Input: part model. Units: mm. Frame: model coordinates. A direction names the side the tool comes from. Round coordinates to 2 decimals unless told otherwise and drop trailing zeros. Loops run counter-clockwise (first coordinate to the right, second up) from the corner with the lowest first, then second, coordinate; pieces in that order, holes last. Notation, with made-up numbers: M 40,45.25 L 52,45.25 A21 ccw 52,84.25 Z; hole C 67,9 d9. An arc over 180 degrees is marked long. Use one line per item in the form item = value. Start each with the question number.
Q1. Section query A-A, the plane x = 0. Output: boundary loops of the cut face in (y, z).
Q2. Section query B-B, the plane z = -44. Output: boundary loops of the cut face in (x, y).
Q3. Section query C-C, the plane x = -18. Output: boundary loops of the cut face in (y, z), and give its area (3 significant figures).
Q4. Access query for faces 1 (the conical face through (64.135, 13.608, -12.544)), 2 (the cylindrical face through (-63.014, 56.359, -12.703)), 3 (the conical face through (61.865, 13.608, -12.544)). Directions: +Z, -Z, +X, -X, +Y, -Y. A direction counts if a zero-diameter tool reaches every point of the face in a straight line with its end or side. Return the directions, or none.
Q5. Section query D-D, the plane x = -33. Output: boundary loops of the cut face in (y, z).
Q6. Mould query, pull axis Z, two halves, no side actions, for faces 4 (the flat face through (-64.5, 35, -43)), 5 (the cylindrical face through (63.02, 17.77, -65.95)), 6 (the conical face through (64.358, 10.775, -72.764)). Classes: pulls with the +Z half, pulls with the -Z half, needs draft (parallel to the pull), parting line crosses it, or undercut.
Q7. Ray query, line 1 along Y through (x, z) = (18, -1); line 2 along X through (y, z) = (45, -48); line 3 along Y through (x, z) = (62, -38). Return the intervals inside material, ascending.
Q8. First-contact query: P1, Ø2.5, axis at y = 52.32, z = -68, coming from the +X side; P2, Ø1, axis at x = 63, y = 39.5, coming from the -Z side; P3, Ø2, axis at x = 63, y = 37, coming from the +Z side; P4, Ø2.5, axis at x = 0, y = 17, coming from the -Z side. Flat tips, straight axial feed; report the tip coordinate or a pass-through.
```python
from build123d import *

# Parameters (mm, degrees)
F_70MM_DEPTH            = 70
FILLET_1_R              = 3
CUT_EXTRUDE_1_REACH     = 170.612
SKETCH_2_R              = 2.05
SKETCH_2_R_2            = 7.5
CUT_EXTRUDE_2_REACH     = 170.612
SKETCH_3_R              = 9.5
SKETCH_4_W              = 18
SKETCH_4_H              = 45
CUT_EXTRUDE_3_DEPTH     = 169.611980594
FILLET_2_R              = 4
FILLET_3_R              = 35
HOLE_WIZARD_3_1_3_1_1_D = 3.1
CHAMFER_1_SIZE          = 0.5


with BuildPart() as part:
    # 草图1 → 宽70mm (new body)
    with BuildSketch(Plane(origin=(0, 0, 0), x_dir=(1, 0, 0), z_dir=(0, 1, 0))):
        Polygon((-64.5, 0), (64.5, 0), (64.5, 83), (61.5, 83), (61.5, 3), (-61.5, 3), (-61.5, 83), (-64.5, 83), align=None)
    extrude(amount=F_70MM_DEPTH)

    # 圆角1
    fillet_1_edges = [part.edges().sort_by_distance(p)[0] for p in [
        (64.5, 35, 0),
        (-64.5, 35, 0),
        (-61.5, 35, -3),
        (61.5, 35, -3),
    ]]
    fillet(fillet_1_edges, radius=FILLET_1_R)

    # 草图2 → 切除-拉伸1 (cut, up to next)
    with BuildSketch(Plane(origin=(64.5, 0, 0), x_dir=(0, 0, -1), z_dir=(1, 0, 0)), mode=Mode.PRIVATE) as cut_extrude_1_sk1:
        with Locations((38, 35)):
            Circle(SKETCH_2_R)
    cut_extrude_1_tool1 = extrude(cut_extrude_1_sk1.sketch, amount=-CUT_EXTRUDE_1_REACH, mode=Mode.PRIVATE) & part.part
    # 草图2 → 切除-拉伸1 (cut, up to next)
    with BuildSketch(Plane(origin=(64.5, 0, 0), x_dir=(0, 0, -1), z_dir=(1, 0, 0)), mode=Mode.PRIVATE) as cut_extrude_1_sk2:
        with Locations((68, 52.320508076)):
            Circle(SKETCH_2_R)
    cut_extrude_1_tool2 = extrude(cut_extrude_1_sk2.sketch, amount=-CUT_EXTRUDE_1_REACH, mode=Mode.PRIVATE) & part.part
    # 草图2 → 切除-拉伸1 (cut, up to next)
    with BuildSketch(Plane(origin=(64.5, 0, 0), x_dir=(0, 0, -1), z_dir=(1, 0, 0)), mode=Mode.PRIVATE) as cut_extrude_1_sk3:
        with Locations((68, 17.679491924)):
            Circle(SKETCH_2_R)
    cut_extrude_1_tool3 = extrude(cut_extrude_1_sk3.sketch, amount=-CUT_EXTRUDE_1_REACH, mode=Mode.PRIVATE) & part.part
    # 草图2 → 切除-拉伸1 (cut, up to next)
    with BuildSketch(Plane(origin=(64.5, 0, 0), x_dir=(0, 0, -1), z_dir=(1, 0, 0)), mode=Mode.PRIVATE) as cut_extrude_1_sk4:
        with Locations((58, 35)):
            Circle(SKETCH_2_R_2)
    cut_extrude_1_tool4 = extrude(cut_extrude_1_sk4.sketch, amount=-CUT_EXTRUDE_1_REACH, mode=Mode.PRIVATE) & part.part
    add(cut_extrude_1_tool1.solids().sort_by_distance((64.5, 35, -38))[0], mode=Mode.SUBTRACT)
    add(cut_extrude_1_tool2.solids().sort_by_distance((64.5, 52.320508, -68))[0], mode=Mode.SUBTRACT)
    add(cut_extrude_1_tool3.solids().sort_by_distance((64.5, 17.679492, -68))[0], mode=Mode.SUBTRACT)
    add(cut_extrude_1_tool4.solids().sort_by_distance((64.5, 35, -58))[0], mode=Mode.SUBTRACT)

    # 草图3 → 切除-拉伸2 (cut, up to next)
    with BuildSketch(Plane.ZY.offset(64.5), mode=Mode.PRIVATE) as cut_extrude_2_sk1:
        with Locations((-58, 35)):
            Circle(SKETCH_3_R)
    cut_extrude_2_tool1 = extrude(cut_extrude_2_sk1.sketch, amount=-CUT_EXTRUDE_2_REACH, mode=Mode.PRIVATE) & part.part
    add(cut_extrude_2_tool1.solids().sort_by_distance((-64.5, 35, -58))[0], mode=Mode.SUBTRACT)

    # 草图4 → 切除-拉伸3 (cut, through all)
    with BuildSketch(Plane(origin=(64.5, 0, 0), x_dir=(0, 0, -1), z_dir=(1, 0, 0))):
        with Locations((20.5, 35)):
            Rectangle(SKETCH_4_W, SKETCH_4_H)
    extrude(amount=-CUT_EXTRUDE_3_DEPTH, mode=Mode.SUBTRACT)

    # 圆角2
    fillet_2_edges = [part.edges().sort_by_distance(p)[0] for p in [
        (63, 57.5, -29.5),
        (-63, 57.5, -29.5),
        (63, 12.5, -29.5),
        (-63, 12.5, -29.5),
        (63, 12.5, -11.5),
        (-63, 12.5, -11.5),
        (63, 57.5, -11.5),
        (-63, 57.5, -11.5),
    ]]
    fillet(fillet_2_edges, radius=FILLET_2_R)

    # 圆角3
    fillet_3_edges = [part.edges().sort_by_distance(p)[0] for p in [
        (63, 70, -83),
        (-63, 70, -83),
        (-63, 0, -83),
        (63, 0, -83),
    ]]
    fillet(fillet_3_edges, radius=FILLET_3_R - 0.0001)  # a hair under: the kernel refuses the full size

    # Ø3.1 (3.1) 直径孔1 (through all)
    with Locations(Plane(origin=(0, 53, -3), x_dir=(-1, 0, 0), z_dir=(0, 0, -1))):
        with Locations((0, 0), (-18, -18), (0, -36), (18, -18)):
            Hole(HOLE_WIZARD_3_1_3_1_1_D / 2)

    # 倒角1
    chamfer_1_edges = [part.edges().sort_by_distance(p)[0] for p in [
        (-64.5, 35, -29.5),
        (-61.5, 35, -29.5),
        (-64.5, 35, -11.5),
        (-61.5, 35, -11.5),
        (-64.5, 12.5, -20.5),
        (-61.5, 12.5, -20.5),
        (64.5, 35, -29.5),
        (61.5, 35, -29.5),
        (64.5, 12.5, -20.5),
        (61.5, 12.5, -20.5),
        (64.5, 57.5, -20.5),
        (61.5, 57.5, -20.5),
        (64.5, 35, -11.5),
        (61.5, 35, -11.5),
        (-61.5, 56.328427125, -28.328427125),
        (-64.5, 56.328427125, -28.328427125),
        (-61.5, 56.328427125, -12.671572875),
        (-64.5, 56.328427125, -12.671572875),
        (-61.5, 13.671572875, -28.328427125),
        (-64.5, 13.671572875, -28.328427125),
        (-61.5, 13.671572875, -12.671572875),
        (-64.5, 13.671572875, -12.671572875),
        (64.5, 13.671572875, -28.328427125),
        (61.5, 13.671572875, -28.328427125),
        (64.5, 56.328427125, -28.328427125),
        (61.5, 56.328427125, -28.328427125),
        (64.5, 13.671572875, -12.671572875),
        (61.5, 13.671572875, -12.671572875),
        (64.5, 56.328427125, -12.671572875),
        (61.5, 56.328427125, -12.671572875),
        (61.5, 70, -27.00005),
        (-64.5, 70, -25.50005),
        (61.5, 0, -27.00005),
        (61.5, 10.251233369, -72.748766631),
        (61.5, 59.748766631, -72.748766631),
        (64.5, 10.251233369, -72.748766631),
        (64.5, 59.748766631, -72.748766631),
        (-64.5, 0, -25.50005),
        (-64.5, 10.251233369, -72.748766631),
        (-64.5, 59.748766631, -72.748766631),
        (-61.5, 10.251233369, -72.748766631),
        (-61.5, 59.748766631, -72.748766631),
        (64.5, 0, -25.50005),
        (64.5, 70, -25.50005),
        (0, 0, 0),
        (-61.5, 0, -27.00005),
        (0, 0, -3),
        (-63.621320344, 0, -0.878679656),
        (63.621320344, 0, -0.878679656),
        (0, 70, 0),
        (0, 70, -3),
        (-61.5, 70, -27.00005),
        (-63.621320344, 70, -0.878679656),
        (63.621320344, 70, -0.878679656),
        (-60.621320344, 0, -3.878679656),
        (-60.621320344, 70, -3.878679656),
        (60.621320344, 0, -3.878679656),
        (60.621320344, 70, -3.878679656),
        (-64.5, 57.5, -20.5),
        (-61.5, 57.5, -20.5),
    ]]
    chamfer(chamfer_1_edges, length=CHAMFER_1_SIZE)


solid = part.part
```
Results found:
q1.outline = M 0,-2.5 L 0.5,-3 L 15.45,-3 L 15.45,0 L 0.5,0 L 0,-0.5 Z; M 18.55,-3 L 51.45,-3 L 51.45,0 L 18.55,0 Z; M 54.55,-3 L 69.5,-3 L 70,-2.5 L 70,-0.5 L 69.5,0 L 54.55,0 Z
q2.outline = M -64.5,0.5 L -64,0 L -62,0 L -61.5,0.5 L -61.5,69.5 L -62,70 L -64,70 L -64.5,69.5 Z; M 61.5,0.5 L 62,0 L 64,0 L 64.5,0.5 L 64.5,69.5 L 64,70 L 62,70 L 61.5,69.5 Z
q3.outline = M 0,-2.5 L 0.5,-3 L 33.45,-3 L 33.45,0 L 0.5,0 L 0,-0.5 Z; M 36.55,-3 L 69.5,-3 L 70,-2.5 L 70,-0.5 L 69.5,0 L 36.55,0 Z
q3.area = 200 mm²
q4.face_1 = +X
q4.face_2 = +X, -X
q4.face_3 = none
q5.outline = M 0,-2.5 L 0.5,-3 L 69.5,-3 L 70,-2.5 L 70,-0.5 L 69.5,0 L 0.5,0 L 0,-0.5 Z
q6.face_4 = needs draft
q6.face_5 = undercut
q6.face_6 = pulls with the -Z half
q7.line_1 = 0 to 33.45, 36.55 to 70
q7.line_2 = -64.5 to -61.5, 61.5 to 64.5
q7.line_3 = 0 to 32.95, 37.05 to 70
q8.P1 = -61.5
q8.P2 = -82.77
q8.P3 = -0.04
q8.P4 = through
